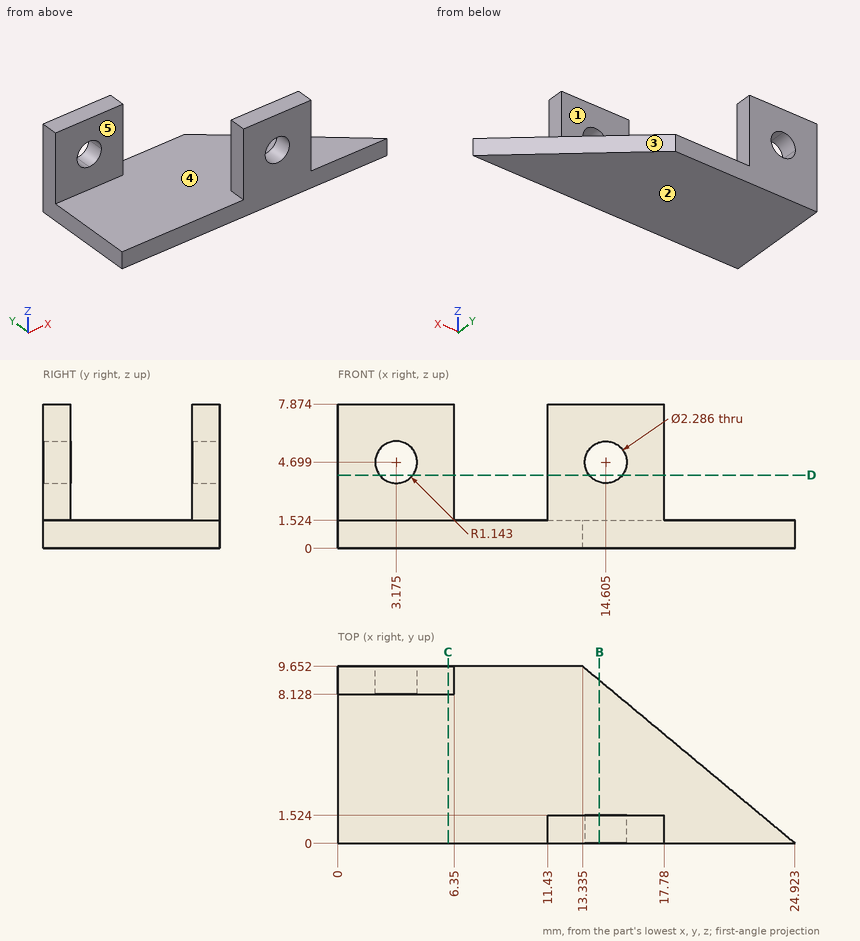
Could you check a few things on this drawing? It's one solid part, dimensions in mm from its lowest x, y, z. A direction names the side the tool comes from. Give positions to 0.01 mm unless a question says otherwise; leave off trailing zeros. Write each loop counter-clockwise with the first axis right and the second up, starting at its lowest first coordinate (ties: lowest second). Pieces come first, ordered by that corner, then holes. Notation, with made-up numbers: (0.25, 22) - (8.25, 22) arc R15 ccw to (8.25, 50) - close; hole circle Ø8 at (-4, 31.5). An arc over 180 degrees is marked (long way). Use CSV: the item, a comma, the result in double quotes. Start each with the question number.
Item 1: I want a section at B-B, the plane x = 14.25. Please give me the cut outline in (y, z) (1 decimal), then the cut area to 3 significant figures.
Item 2: If we mould it in two halves opening along Y, with no side actions, what happens to the marked faces 3, 4 and 5? For each: pulls with the +Y half, pulls with the -Y half, needs draft (parallel to the pull), parting line crosses it, or undercut.
Item 3: I want a section at D-D, the plane z = 4. Give the number of separate pieces and of enclosed holes in the cut face.
Item 4: I'm going to push flat-ended pins straight in: pin 1 (2 mm diameter, centred on x = 4, y = 3.5, fed in from -Z); pin 2 (3.5 mm diameter, centred on x = 14.605, z = 4.699, fed in from +Y); pin 3 (1.7 mm diameter, centred on y = 0.5, z = 3.5, fed in from -X); pin 4 (1.7 mm diameter, centred on y = 8.5, z = 6, fed in from +X). Where does each tip first touch, or does it pass through?
Item 5: If I drill on line 1 along Z through (x, y) = (7, 0.5) (1 decimal); line 2 along X through (y, z) = (9, 2.75), over which ranges is the centre line in solid material (lowest first)?
Item 6: For the marked faces 1 and 2, which set-ups out of +Z, -Z, +X, -X, +Y, -Y let a thin tool reach every point of the face, with its end or its side?
Item 7: I want a section at C-C, the plane x = 6. Please give me the cut outline in (y, z) (1 decimal), then the cut area to 3 significant figures.
Findings:
1,outline,"(0, 0) - (8.9, 0) - (8.9, 1.5) - (1.5, 1.5) - (1.5, 3.6) - (0, 3.6) - close; (0, 5.8) - (1.5, 5.8) - (1.5, 7.9) - (0, 7.9) - close"
1,area,"19.9 mm2"
2,face 3,"pulls with the +Y half"
2,face 4,"needs draft"
2,face 5,"pulls with the -Y half"
3,separate pieces,"4"
3,enclosed holes,"0"
4,pin 1,"stops at z = 0"
4,pin 2,"stops at y = 1.52"
4,pin 3,"stops at x = 11.43"
4,pin 4,"stops at x = 6.35"
5,line 1,"z = 0 to 1.5"
5,line 2,"x = 0 to 6.35"
6,face 1,"+Z, +X, -X, +Y"
6,face 2,"-Z, +X, -X, +Y, -Y"
7,outline,"(0, 0) - (9.7, 0) - (9.7, 7.9) - (8.1, 7.9) - (8.1, 1.5) - (0, 1.5) - close"
7,area,"24.4 mm2"
